Here's how the part is built. I have some questions about the finished solid (model axes, mm). A direction names the side the tool comes from. Coordinates: 2 decimals unless noted, no trailing zeros. Loops run counter-clockwise (first coordinate to the right, second up) from the corner with the lowest first, then second, coordinate; pieces in that order, holes last. Notation, with made-up numbers: (59.25, -3) -> (79.25, -3) arc R34 cw to (79.25, 33) -> close; hole circle Ø10 at (38.25, 23). An arc over 180 degrees is marked (long way). Answer as a JSON object with one key per item and string values. Group by question number.
Q1. I'm going to push flat-ended pins straight in: pin 1 (0.7 mm diameter, centred on y = 12, z = -1.5, fed in from +X); pin 2 (1 mm diameter, centred on x = 0, y = 4.5, fed in from +Z); pin 3 (1 mm diameter, centred on x = -2.5, y = 2.5, fed in from -Z); pin 4 (1 mm diameter, centred on y = 8, z = 3, fed in from -X). Where does each tip first touch, or does it pass through?
Q2. I want a section at A-A on y = 9.75. Write out the boundary of the cut face in (x, z).
Q3. I want a section at B-B on y = 4. Write out the boundary of the cut face in (x, z).
Q4. On a 3-axis mill with a long thin cutter (end or side, diameter ignored), from which of +Z, -Z, +X, -X, +Y, -Y can I reach the whole of each face in a straight line? I mean faces 4 (the cylindrical face through (4.624, 10.08, 1.027)), 5 (the flat face through (2, 9.525, 2)). Say none if no direction works.
Q5. Thinking about a two-plate mould opening in Z: for faces 1 (the flat face through (0, 11.938, 0)), 2 (the flat face through (0, 0, 0)), 3 (the cylindrical face through (1.468, 4.829, 1.915)), which applies, released by +Z, released by -Z, zero draft, split by the parting line, or undercut?
Q6. I need wall thicknesses on line 1 (Y direction, x = -2, z = -1.5) (3 decimals); line 2 (Z direction, x = 0.5, y = 7.5); line 3 (Z direction, x = -2.75, y = 10.75). Which ranges of each line are inside material? Lowest first, please.
```python
from build123d import *

# Parameters (mm, degrees)
CUT_EXTRUDE1_DEPTH = 0.635
CIRPATTERN1_COUNT  = 4


with BuildPart() as part:
    # Sketch1 → Revolve1 (revolve)
    with BuildSketch(Plane.XY, mode=Mode.PRIVATE) as revolve1_sk:
        with BuildLine():
            Line((0, 0), (2.413, 0))
            Line((2.413, 0), (2.413, 9.525))
            Line((2.413, 9.525), (4.7371, 9.525))
            Line((4.7371, 9.525), (4.7371, 10.618743367))
            ThreePointArc((4.7371, 10.618743367), (2.548065575, 12.067962924), (0, 12.7))
            Line((0, 12.7), (0, 0))
        make_face()
    revolve(revolve1_sk.sketch.rotate(Axis((0, 0, 0), (0, 1, 0)), 90), axis=Axis((0, 0, 0), (0, 1, 0)))

    # Sketch2 → Cut-Extrude1 (cut, symmetric)
    with BuildSketch(Plane.XY):
        with BuildLine():
            Line((0, 11.938), (2.828492677, 11.938))
            ThreePointArc((2.828492677, 11.938), (1.450712269, 12.454359079), (0, 12.7))
            Line((0, 12.7), (0, 11.938))
        make_face()
    cut_extrude1 = extrude(amount=CUT_EXTRUDE1_DEPTH, both=True, mode=Mode.SUBTRACT)

    # CirPattern1: Cut-Extrude1 ×4 about axis
    cirpattern1_axis = Axis((0, 0, 0), (0, 1, 0))
    for i in range(1, CIRPATTERN1_COUNT):
        add(cut_extrude1.rotate(cirpattern1_axis, i * 360 / CIRPATTERN1_COUNT), mode=Mode.SUBTRACT)


solid = part.part
```
Result set:
{
 "1": {"pin 1": "stops at x = 3.03", "pin 2": "stops at z = 2.41", "pin 3": "stops at z = -1.35", "pin 4": "passes through"},
 "2": {"outline": "circle Ø9.47 at (0, 0)"},
 "3": {"outline": "circle Ø4.83 at (0, 0)"},
 "4": {"face 4": "+Y, -Y", "face 5": "-Y"},
 "5": {"face 1": "undercut", "face 2": "zero draft", "face 3": "split by the parting line"},
 "6": {"line 1": "y = 9.525 to 12.089", "line 2": "z = -2.36 to 2.36", "line 3": "z = -3.68 to 3.68"}
}
